The listing builds one solid part. Answer for the finished solid, in the listing's coordinates (mm). A direction names the side the tool comes from. Round coordinates to 2 decimals unless told otherwise and drop trailing zeros. Loops run counter-clockwise (first coordinate to the right, second up) from the corner with the lowest first, then second, coordinate; pieces in that order, holes last. Notation, with made-up numbers: (12, 11.5) - (51, 11.5) arc R25 cw to (51, 29.5) - close; hole circle Ø4 at (15, 69). An arc over 180 degrees is marked (long way). Write item = value, one per line. Start each with the question number.
1) Section A-A, the plane z = 7 is taken. Determine the outline of the cut face in (x, y), and give its area (3 significant figures).
2) Section D-D, the plane x = -2.25 is taken. Determine the outline of the cut face in (y, z).
3) A tool of negligible diameter and unlimited length cuts with its end or side. For faces 1 (the cylindrical face through (4, 2, 3)), 2 (the flat face through (-2.5, 2, 7)), 3 (the flat face through (-4.7, 2.5, -5.6)), from which of +Z, -Z, +X, -X, +Y, -Y can it reach the whole face along a straight path? Write none if from no direction.
4) Straight lines are drawn through the part: line 1 along X through (y, z) = (1.2, 7); line 2 along X through (y, z) = (2.65, -3.25); line 3 along Z through (x, y) = (1.25, 0.6). For each, find the intervals that lie inside material, in ascending order.
5) Given pin 1 Ø1.7 at (y, z) = (2.5, 6.5) entering from -X; pin 2 Ø5 at (x, z) = (6.06, -3.5) entering from -Y; pin 3 Ø1 at (y, z) = (3, 7) entering from +X; pin 4 Ø3 at (x, y) = (2.5, 3.5) entering from -Z, each flat-ended and moving along its own axis, determine where each tip first touches the part or whether it passes through.
6) For a pull along Z with two mould halves and no side action, classify faces 4 (the cylindrical face through (-2.55, 2.46, -4.53)), 5 (the cylindrical face through (-9.314, 2.535, -3.012)), 6 (the flat face through (0, 2, 10)), 7 (the cylindrical face through (-0.596, 2.535, 2.685)) as released by +Z, released by -Z, zero draft, split by the parting line, or undercut.
7) Section B-B, the plane x = 0 is taken. Determine the outline of the cut face in (y, z), and give its area (3 significant figures).
8) Section C-C, the plane z = -3.5 is taken. Determine the outline of the cut face in (x, y).
from build123d import *

# Parameters (mm, degrees)
SKETCH1_R                = 5
BOSS_EXTRUDE1_DEPTH      = 5
SKETCH2_W                = 5
SKETCH2_H                = 10
BOSS_EXTRUDE2_DEPTH      = 5
SKETCH3_R                = 1.5
CUT_EXTRUDE1_DEPTH       = 6
FILLET1_R                = 1.5
CIRPATTERN1_COUNT        = 3
FILLET1_OF_CIRPATTERN1_R = 1.5
SKETCH4_R                = 2.75
CUT_EXTRUDE2_DEPTH       = 6


with BuildPart() as part:
    # Sketch1 → Boss-Extrude1 (new body)
    with BuildSketch(Plane(origin=(0, 0, 0), x_dir=(1, 0, 0), z_dir=(0, 1, 0))):
        Circle(SKETCH1_R)
    extrude(amount=BOSS_EXTRUDE1_DEPTH)

    # Sketch2 → Boss-Extrude2 (add)
    with BuildSketch(Plane(origin=(0, 0, 0), x_dir=(1, 0, 0), z_dir=(0, 1, 0))):
        with Locations((0, -5)):
            Rectangle(SKETCH2_W, SKETCH2_H)
    boss_extrude2 = extrude(amount=BOSS_EXTRUDE2_DEPTH)

    # Sketch3 → Cut-Extrude1 (cut, through all)
    with BuildSketch(Plane(origin=(0, 5, 0), x_dir=(1, 0, 0), z_dir=(0, 1, 0))):
        with Locations((0, -7)):
            Circle(SKETCH3_R)
    cut_extrude1 = extrude(amount=-CUT_EXTRUDE1_DEPTH, mode=Mode.SUBTRACT)

    # Fillet1
    fillet1_edges = [part.edges().sort_by_distance(p)[0] for p in [
        (2.5, 2.5, 4.330127019),
        (2.5, 2.5, 10),
        (-2.5, 2.5, 4.330127019),
        (-2.5, 2.5, 10),
    ]]
    fillet(fillet1_edges, radius=FILLET1_R)

    # CirPattern1: Boss-Extrude2, Cut-Extrude1 ×3 about axis
    cirpattern1_axis = Axis((0, 0, 0), (0, 1, 0))
    for i in range(1, CIRPATTERN1_COUNT):
        add(boss_extrude2.rotate(cirpattern1_axis, i * 360 / CIRPATTERN1_COUNT))
        add(cut_extrude1.rotate(cirpattern1_axis, i * 360 / CIRPATTERN1_COUNT), mode=Mode.SUBTRACT)

    # Fillet1 of CirPattern1
    fillet1_of_cirpattern1_edges = [part.edges().sort_by_distance(p)[0] for p in [
        (2.5, 2.5, -4.330127019),
        (7.410254038, 2.5, -7.165063509),
        (5, 2.5, 0),
        (9.910254038, 2.5, -2.834936491),
        (-5, 2.5, 0),
        (-9.910254038, 2.5, -2.834936491),
        (-2.5, 2.5, -4.330127019),
        (-7.410254038, 2.5, -7.165063509),
    ]]
    fillet(fillet1_of_cirpattern1_edges, radius=FILLET1_OF_CIRPATTERN1_R)

    # Sketch4 → Cut-Extrude2 (cut, through all)
    with BuildSketch(Plane(origin=(0, 5, 0), x_dir=(1, 0, 0), z_dir=(0, 1, 0))):
        Circle(SKETCH4_R)
    extrude(amount=-CUT_EXTRUDE2_DEPTH, mode=Mode.SUBTRACT)


solid = part.part
Geometry check:
q1.outline = (-2.5, 0) - (-1.5, 0) - (-1.5, 5) - (-2.5, 5) - close; (1.5, 0) - (2.5, 0) - (2.5, 5) - (1.5, 5) - close
q1.area = 10.0 mm2
q2.outline = (0, -4.54) - (5, -4.54) - (5, -1.58) - (0, -1.58) - close; (0, 1.58) - (5, 1.58) - (5, 9.33) - (0, 9.33) - close
q3.face_1 = +Z, +X, +Y, -Y
q3.face_2 = +Z, -X, +Y, -Y
q3.face_3 = -Z, +Y, -Y
q4.line_1 = -2.5 to -1.5, 1.5 to 2.5
q4.line_2 = -9.36 to -7.54, -4.58 to 4.58, 7.54 to 9.36
q4.line_3 = -4.84 to -2.45, 2.45 to 6.17, 7.83 to 9.98
q5.pin_1 = -2.5
q5.pin_2 = 0
q5.pin_3 = 2.5
q5.pin_4 = -5.2
q6.face_4 = released by -Z
q6.face_5 = split by the parting line
q6.face_6 = released by +Z
q6.face_7 = undercut
q7.outline = (0, -5) - (5, -5) - (5, -2.75) - (0, -2.75) - close; (0, 2.75) - (5, 2.75) - (5, 5.5) - (0, 5.5) - close; (0, 8.5) - (5, 8.5) - (5, 10) - (0, 10) - close
q7.area = 32.5 mm2
q8.outline = (-9.36, 0) - (-7.56, 0) - (-7.56, 5) - (-9.36, 5) - close; (-4.56, 0) - (4.56, 0) - (4.56, 5) - (-4.56, 5) - close; (7.56, 0) - (9.36, 0) - (9.36, 5) - (7.56, 5) - close
